```python
from build123d import *

# Parameters (mm, degrees)
F0_R     = 51.4953011057
F1_DEPTH = 203.2
F2_R     = 20.32
F3_DEPTH = 50.8
F4_R     = 20.32


with BuildPart() as f1:
    # F0 (on Top) → F1 (new body)
    with BuildSketch(Plane.XY):
        Circle(F0_R)
    extrude(amount=F1_DEPTH)

    # F2
    f2_edges = [f1.edges().sort_by_distance(p)[0] for p in [
        (-51.495301, 0, 0),
        (-51.495301, 0, 203.2),
    ]]
    fillet(f2_edges, radius=F2_R)

    # F3 (add): a face of the model
    f3_faces = [f1.faces().sort_by_distance(p)[0] for p in [
        (0, 0, 203.2),
    ]]
    extrude(f3_faces, amount=F3_DEPTH)

    # F4
    f4_edges = [f1.edges().sort_by_distance(p)[0] for p in [
        (-31.175301, 0, 254),
    ]]
    fillet(f4_edges, radius=F4_R)


solid = f1.part
```
Model file for the job. Use its own axes, mm. A direction names the side the tool comes from. Give positions to 0.01 mm unless a question says otherwise; leave off trailing zeros. Write each loop counter-clockwise with the first axis right and the second up, starting at its lowest first coordinate (ties: lowest second). Pieces come first, ordered by that corner, then holes. Notation, with made-up numbers: M -20,-24 L 30,-24 A11 ccw 30,-12 Z; hole C 55,-36 d4. An arc over 180 degrees is marked long. Use a Markdown table: item, result.
1) Tool access for faces 1 (the flat face through (0, 0, 0)), 2 (the cylindrical face through (28.8, -11.94, 218.23)): list every direction of +Z, -Z, +X, -X, +Y, -Y with a clear straight run to the whole face (end or side of a thin tool).
Responses:
| item | result |
|---|---|
| face 1 | -Z, +X, -X, +Y, -Y |
| face 2 | +Z |
2) Pin check, flat tips, straight feed: pin 1 (12 mm diameter, centred on y = -9, z = 193, fed in from +X); pin 2 (1 mm diameter, centred on y = -28.5, z = 152.5, fed in from +X); pin 3 (6 mm diameter, centred on x = -2.5, y = -9, fed in from -Z); pin 4 (3 mm diameter, centred on y = -19.5, z = 80, fed in from +X). Stop position of each tip, or through.
Responses:
| item | result |
|---|---|
| pin 1 | stops at x = 50.54 |
| pin 2 | stops at x = 43.22 |
| pin 3 | stops at z = 0 |
| pin 4 | stops at x = 48.25 |
3) Cut at A-A (z = 156.5). List the corners of the cut face in (x, y), and give its area (3 significant figures).
Responses:
| item | result |
|---|---|
| outline | C 0,0 d102.99 |
| area | 8,330 mm2 |
4) Drill centre lines: line 1 (Y direction, x = -41, z = 142); line 2 (Y direction, x = 0, z = 44.5); line 3 (Z direction, x = 36, y = 5). Where is each one in solid material? Low to high. Write a range as from..to.
Responses:
| item | result |
|---|---|
| line 1 | y = -31.16..31.16 |
| line 2 | y = -51.5..51.5 |
| line 3 | z = 0.67..202.53 |
